from build123d import *

# Parameters (mm, degrees)
SKETCH4_W                = 24
SKETCH4_H                = 27
BOSS_EXTRUDE3_DEPTH      = 3
BOSS_EXTRUDE3_DEPTH_BACK = 8
SKETCH5_W                = 28.405044576
SKETCH5_H                = 3.736732925
SKETCH6_R                = 5
CUT_EXTRUDE1_DEPTH       = 4
CUT_EXTRUDE1_DEPTH_BACK  = 8
SKETCH7_W                = 24
SKETCH7_H                = 27
CUT_EXTRUDE2_DEPTH       = 6
SKETCH8_R                = 1.15
CUT_EXTRUDE3_DEPTH       = 5.0000001
CUT_EXTRUDE4_START       = -2
SKETCH9_R                = 1.9
CUT_EXTRUDE4_DEPTH       = 2


with BuildPart() as part:
    # Sketch4 → Boss-Extrude3 (new body, two sides)
    with BuildSketch(Plane(origin=(0, 0, 0), x_dir=(1, 0, 0), z_dir=(0, 1, 0))) as boss_extrude3_sk:
        Rectangle(SKETCH4_W, SKETCH4_H)
    extrude(amount=BOSS_EXTRUDE3_DEPTH)
    extrude(boss_extrude3_sk.sketch, amount=-BOSS_EXTRUDE3_DEPTH_BACK)

    # Sketch5 → Cut-Revolve1 (revolve, cut)
    with BuildSketch(Plane(origin=(0, 0, 0), x_dir=(0, 0, -1), z_dir=(1, 0, 0))):
        with Locations((0.702522288, -8.868366462)):
            Rectangle(SKETCH5_W, SKETCH5_H)
    revolve(axis=Axis((0, 62, 13.5), (0, 0, -1)), mode=Mode.SUBTRACT)

    # Sketch6 → Cut-Extrude1 (cut, two sides)
    with BuildSketch(Plane(origin=(0, 0, 0), x_dir=(1, 0, 0), z_dir=(0, 1, 0))) as cut_extrude1_sk:
        Circle(SKETCH6_R)
    extrude(amount=CUT_EXTRUDE1_DEPTH, mode=Mode.SUBTRACT)
    extrude(cut_extrude1_sk.sketch, amount=-CUT_EXTRUDE1_DEPTH_BACK, mode=Mode.SUBTRACT)

    # Sketch7 → Cut-Extrude2 (cut)
    with BuildSketch(Plane(origin=(0, 3, 0), x_dir=(1, 0, 0), z_dir=(0, 1, 0))):
        Rectangle(SKETCH7_W, SKETCH7_H)
    extrude(amount=-CUT_EXTRUDE2_DEPTH, mode=Mode.SUBTRACT)

    # Sketch8 → Cut-Extrude3 (cut, through all)
    with BuildSketch(Plane(origin=(0, -3, 0), x_dir=(1, 0, 0), z_dir=(0, 1, 0))):
        with Locations((-10, 6.5)):
            Circle(SKETCH8_R)
        with Locations((-10, -6.5)):
            Circle(SKETCH8_R)
        with Locations((10, -6.5)):
            Circle(SKETCH8_R)
        with Locations((10, 6.5)):
            Circle(SKETCH8_R)
    extrude(amount=-CUT_EXTRUDE3_DEPTH, mode=Mode.SUBTRACT)

    # Sketch9 → Cut-Extrude4 (cut)
    with BuildSketch(Plane(origin=(0, -3, 0), x_dir=(1, 0, 0), z_dir=(0, 1, 0)).offset(CUT_EXTRUDE4_START)):
        with Locations((-10, 6.5)):
            Circle(SKETCH9_R)
        with Locations((-10, -6.5)):
            Circle(SKETCH9_R)
        with Locations((10, -6.5)):
            Circle(SKETCH9_R)
        with Locations((10, 6.5)):
            Circle(SKETCH9_R)
    extrude(amount=-CUT_EXTRUDE4_DEPTH, mode=Mode.SUBTRACT)


solid = part.part
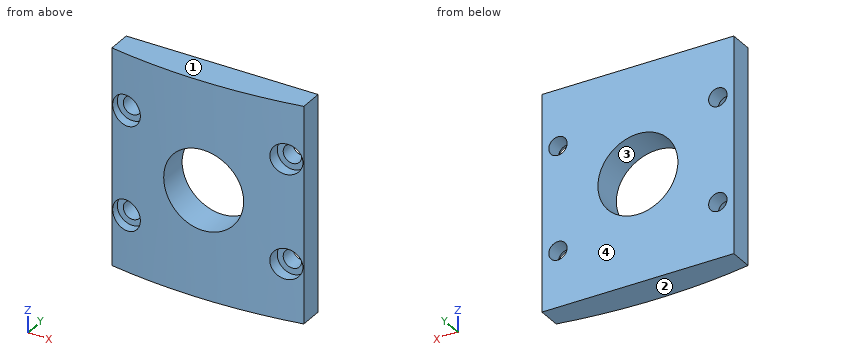
Input: part model. Units: mm. Frame: model coordinates. Face numbers are marked on the shaded views. Round coordinates to 2 decimals unless told otherwise and drop trailing zeros. Write each loop counter-clockwise with the first axis right and the second up, starting at its lowest first coordinate (ties: lowest second). Pieces come first, ordered by that corner, then holes.
1) Draft query along Z for the marked faces 1, 2, 3 and 4. Return one class per face: pulls with the +Z half, pulls with the -Z half, needs draft (parallel to the pull), parting line crosses it, or undercut.
2) Cut plane C-C (z = -1.75). Return the cut outline in (x, y).
3) Cut plane B-B (y = -3.5). Return the cut outline in (x, z).
4) Cut plane A-A (x = 0). Return the cut outline in (y, z), then the cut area to 3 significant figures.
5) Cut plane D-D (x = 10). Return the cut outline in (y, z).
6) Ray query, L1, parallel to Z at x = 10, y = -5.7; L2, parallel to Z at x = -10, y = -4.4; L3, parallel to X at y = -4.5, z = -5.5. Return the intervals inside material, ascending.
7) Contact query for flat-ended pins moving along their axis: P1, Ø2, axis at x = 10, z = 6.5, coming from the -Y side; P2, Ø1.1, axis at x = -11, z = 6.5, coming from the -Y side; P3, Ø5, axis at x = 10, z = -6.5, coming from the -Y side; P4, Ø3, axis at x = -10.5, z = -7, coming from the -Y side. Output: stop coordinate, or through.
Geometry says:
1. face 1: pulls with the +Z half
1. face 2: pulls with the -Z half
1. face 3: undercut
1. face 4: needs draft
2. outline: (-12, -5.95) arc R69 ccw to (-4.68, -6.84) - (-4.68, -3) - (-12, -3) - close; (4.68, -6.84) arc R69 ccw to (12, -5.95) - (12, -3) - (4.68, -3) - close
3. outline: (-12, -13.5) - (12, -13.5) - (12, 13.5) - (-12, 13.5) - close; hole circle Ø2.3 at (-10, -6.5); hole circle Ø2.3 at (-10, 6.5); hole circle Ø10 at (0, 0); hole circle Ø2.3 at (10, -6.5); hole circle Ø2.3 at (10, 6.5)
4. outline: (-7, -13.5) - (-3, -13.5) - (-3, -5) - (-7, -5) - close; (-7, 5) - (-3, 5) - (-3, 13.5) - (-7, 13.5) - close
4. area: 68.0 mm2
5. outline: (-6.27, -13.5) - (-3, -13.5) - (-3, -7.65) - (-5, -7.65) - (-5, -8.4) - (-6.27, -8.4) - close; (-6.27, -4.6) - (-5, -4.6) - (-5, -5.35) - (-3, -5.35) - (-3, 5.35) - (-5, 5.35) - (-5, 4.6) - (-6.27, 4.6) - close; (-6.27, 8.4) - (-5, 8.4) - (-5, 7.65) - (-3, 7.65) - (-3, 13.5) - (-6.27, 13.5) - close
6. L1: z = -13.5 to -8.4, -4.6 to 4.6, 8.4 to 13.5
6. L2: z = -13.5 to -7.65, -5.35 to 5.35, 7.65 to 13.5
6. L3: x = -12 to -10.57, -9.43 to 9.43, 10.57 to 12
7. P1: passes through
7. P2: stops at y = -5
7. P3: stops at y = -6.59
7. P4: stops at y = -6.28
